Can you work these out from the model? Positions are in its coordinate system, mm. Give positions to 0.01 mm unless a question says otherwise; leave off trailing zeros. Loops run counter-clockwise (first coordinate to the right, second up) from the corner with the lowest first, then second, coordinate; pieces in that order, holes last. Notation, with made-up numbers: (-35.5, 27.5) - (-15.5, 27.5) arc R16 cw to (-15.5, 48.5) - close; hole circle Ø2 at (65, -38). An arc over 180 degrees is marked (long way). Use a Markdown table: item, result. Add a question column.
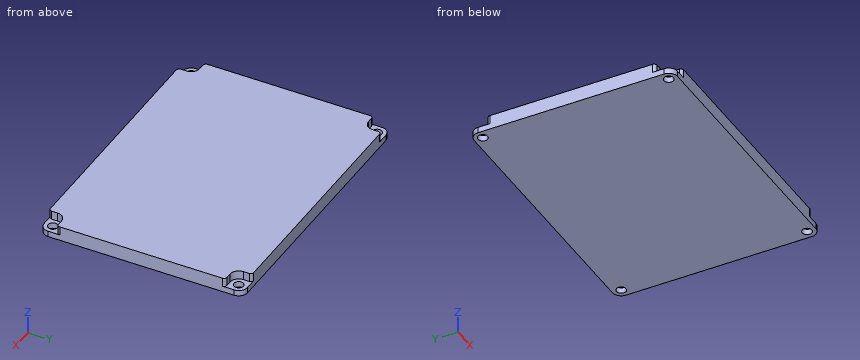
```python
from build123d import *

# Parameters (mm, degrees)
SKETCH_1_W          = 95
SKETCH_1_H          = 70
EXTRUDE_1_DEPTH     = 5
FILLET_1_R          = 3
SKETCH_13_R         = 1.65
CUT_EXTRUDE_2_DEPTH = 5
SKETCH_14_R         = 3
CUT_EXTRUDE_3_DEPTH = 3
CUT_EXTRUDE_4_DEPTH = 3
FILLET_3_R          = 1


with BuildPart() as part:
    # ｽｹｯﾁ1 → ﾎﾞｽ - 押し出し1 (new body)
    with BuildSketch(Plane.XY):
        with Locations((47.5, 35)):
            Rectangle(SKETCH_1_W, SKETCH_1_H)
    extrude(amount=EXTRUDE_1_DEPTH)

    # ﾌｨﾚｯﾄ1
    fillet_1_edges = [part.edges().sort_by_distance(p)[0] for p in [
        (0, 70, 2.5),
        (95, 70, 2.5),
        (95, 0, 2.5),
        (0, 0, 2.5),
    ]]
    fillet(fillet_1_edges, radius=FILLET_1_R)

    # ｽｹｯﾁ13 → ｶｯﾄ - 押し出し2 (cut)
    with BuildSketch(Plane.XY.offset(5)):
        with Locations((3, 67)):
            Circle(SKETCH_13_R)
        with Locations((92, 67)):
            Circle(SKETCH_13_R)
        with Locations((3, 3)):
            Circle(SKETCH_13_R)
        with Locations((92, 3)):
            Circle(SKETCH_13_R)
    extrude(amount=-CUT_EXTRUDE_2_DEPTH, mode=Mode.SUBTRACT)

    # ｽｹｯﾁ14 → ｶｯﾄ - 押し出し3 (cut)
    with BuildSketch(Plane.XY.offset(5)):
        with Locations((3, 67)):
            Circle(SKETCH_14_R)
        with Locations((92, 67)):
            Circle(SKETCH_14_R)
        with Locations((3, 3)):
            Circle(SKETCH_14_R)
        with Locations((92, 3)):
            Circle(SKETCH_14_R)
    extrude(amount=-CUT_EXTRUDE_3_DEPTH, mode=Mode.SUBTRACT)

    # ｽｹｯﾁ15 → ｶｯﾄ - 押し出し4 (cut)
    with BuildSketch(Plane.XY.offset(5)):
        with BuildLine():
            Line((95, 3), (95, 6))
            Line((95, 6), (92, 6))
            ThreePointArc((92, 6), (94.121320344, 5.121320344), (95, 3))
        make_face()
        with BuildLine():
            Line((89, 3), (89, 0))
            Line((89, 0), (92, 0))
            ThreePointArc((92, 0), (89.878679656, 0.878679656), (89, 3))
        make_face()
        with BuildLine():
            Line((6, 0), (6, 3))
            ThreePointArc((6, 3), (5.121320344, 0.878679656), (3, 0))
            Line((3, 0), (6, 0))
        make_face()
        with BuildLine():
            Line((3, 6), (0, 6))
            Line((0, 6), (0, 3))
            ThreePointArc((0, 3), (0.878679656, 5.121320344), (3, 6))
        make_face()
        with BuildLine():
            Line((0, 64), (3, 64))
            ThreePointArc((3, 64), (0.878679656, 64.878679656), (0, 67))
            Line((0, 67), (0, 64))
        make_face()
        with BuildLine():
            ThreePointArc((3, 70), (5.121320344, 69.121320344), (6, 67))
            Line((6, 67), (6, 70))
            Line((6, 70), (3, 70))
        make_face()
        with BuildLine():
            Line((92, 70), (89, 70))
            Line((89, 70), (89, 67))
            ThreePointArc((89, 67), (89.878679656, 69.121320344), (92, 70))
        make_face()
        with BuildLine():
            ThreePointArc((95, 67), (94.121320344, 64.878679656), (92, 64))
            Line((92, 64), (95, 64))
            Line((95, 64), (95, 67))
        make_face()
    extrude(amount=-CUT_EXTRUDE_4_DEPTH, mode=Mode.SUBTRACT)

    # ﾌｨﾚｯﾄ3
    fillet_3_edges = [part.edges().sort_by_distance(p)[0] for p in [
        (0, 64, 3.5),
        (0, 6, 3.5),
        (6, 0, 3.5),
        (89, 0, 3.5),
        (95, 64, 3.5),
        (89, 70, 3.5),
        (6, 70, 3.5),
        (95, 6, 3.5),
    ]]
    fillet(fillet_3_edges, radius=FILLET_3_R)


solid = part.part
```
1. Please list where these lines run through material, in increasing order: line 1 along Y through (x, z) = (3, 1); line 2 along X through (y, z) = (67, 1). Write a range as [from, to].
2. Will these pins go through, and if not, where does the flat tip stop? P1, Ø2, axis at y = 1.5, z = 3.5, coming from the -X side; P2, Ø2, axis at x = 92.5, z = 3.5, coming from the -Y side; P3, Ø2, axis at y = 1.5, z = 4, coming from the +X side; P4, Ø1.5, axis at x = 25, y = 20.5, coming from the -Z side.
3. Suppose I cut it at A-A (z = 2.8). List the corners of the cut face in (x, y) for me.
Results below:
| question | item | result |
|---|---|---|
| 1 | line 1 | [0, 1.35], [4.65, 65.35], [68.65, 70] |
| 1 | line 2 | [0, 1.35], [4.65, 90.35], [93.65, 95] |
| 2 | P1 | x = 6 |
| 2 | P2 | y = 5.96 |
| 2 | P3 | x = 89 |
| 2 | P4 | z = 0 |
| 3 | outline | (0, 7) arc R1 ccw to (1, 6) - (3, 6) arc R3 cw to (6, 3) - (6, 1) arc R1 ccw to (7, 0) - (88, 0) arc R1 ccw to (89, 1) - (89, 3) arc R3 cw to (92, 6) - (94, 6) arc R1 ccw to (95, 7) - (95, 63) arc R1 ccw to (94, 64) - (92, 64) arc R3 cw to (89, 67) - (89, 69) arc R1 ccw to (88, 70) - (7, 70) arc R1 ccw to (6, 69) - (6, 67) arc R3 cw to (3, 64) - (1, 64) arc R1 ccw to (0, 63) - close |
